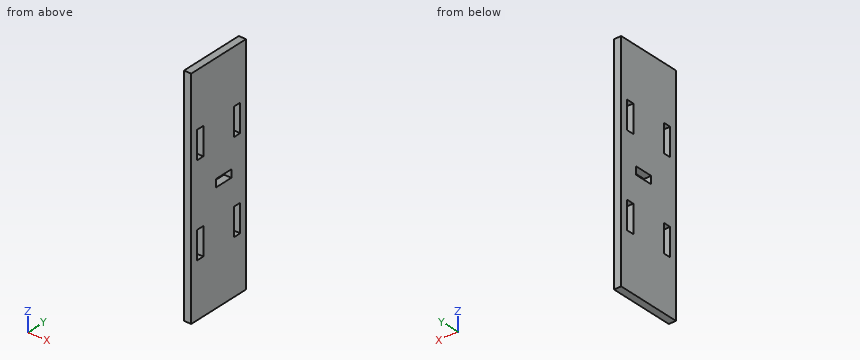
from build123d import *

# Parameters (mm, degrees)
SKETCH1_W           = 685
SKETCH1_H           = 250
BASE_FLANGE1_DEPTH  = 8
SKETCH6_W           = 60
SKETCH6_H           = 8
SKETCH6_W_2         = 70
EXTRUDE1_DEPTH      = 8
SKETCH7_W           = 250
SKETCH7_H           = 73.5
BASE_FLANGE2_DEPTH  = 8
SKETCH12_W          = 30.5
SKETCH12_H          = 8.5
EXTRUDE2_DEPTH      = 699.681794525
SKETCH14_W          = 250
SKETCH14_H          = 8
BASE_FLANGE3_DEPTH  = 50.5
SKETCH19_W          = 60
SKETCH19_H          = 8
SKETCH19_W_2        = 70
EXTRUDE3_DEPTH      = 8
BREAK_CORNER1_START = 41.5
BREAK_CORNER1_DEPTH = 8
EXTRUDE4_DEPTH      = 8
BASE_FLANGE4_DEPTH  = 8
SKETCH38_W          = 8.5
SKETCH38_H          = 20.5
EXTRUDE5_DEPTH      = 10
SKETCH39_W          = 20.5
SKETCH39_H          = 8.5
EXTRUDE6_DEPTH      = 10


# Read off the part's stored shape, not the designer's step: Break-Corner1
# Sheet-metal steps are written as plain solids
with BuildPart() as part:
    # Sketch1 → Base-Flange1 (new body)
    with BuildSketch(Plane(origin=(0, 0, 0), x_dir=(1, 0, 0), z_dir=(0, 1, 0))):
        Rectangle(SKETCH1_W, SKETCH1_H)
    extrude(amount=-BASE_FLANGE1_DEPTH)

    # Sketch6 → Extrude1 (cut)
    with BuildSketch(Plane(origin=(342.5, 0, 0), x_dir=(0, 0, -1), z_dir=(1, 0, 0))):
        with Locations((-95, -4)):
            Rectangle(SKETCH6_W, SKETCH6_H)
        with Locations((95, -4)):
            Rectangle(SKETCH6_W, SKETCH6_H)
        with Locations((0, -4)):
            Rectangle(SKETCH6_W_2, SKETCH6_H)
    extrude1 = extrude(amount=-EXTRUDE1_DEPTH, mode=Mode.SUBTRACT)

    # Mirror1: Extrude1 across plane
    add(extrude1.mirror(Plane(origin=(0, 0, 0), x_dir=(0, 0, 1), z_dir=(1, 0, 0))), mode=Mode.SUBTRACT)

    # Sketch39 → Extrude6 (cut)
    with BuildSketch(Plane.XZ.offset(8)):
        with Locations((289.5, 0)):
            Rectangle(SKETCH39_W, SKETCH39_H)
        with Locations((229.5, 0)):
            Rectangle(SKETCH39_W, SKETCH39_H)
        with Locations((-289.5, 0)):
            Rectangle(SKETCH39_W, SKETCH39_H)
        with Locations((-229.5, 0)):
            Rectangle(SKETCH39_W, SKETCH39_H)
    extrude(amount=-EXTRUDE6_DEPTH, mode=Mode.SUBTRACT)


with BuildPart() as body_2:
    # Sketch7 → Base-Flange2 (new body)
    with BuildSketch(Plane(origin=(334.5, 0, 0), x_dir=(0, 0, -1), z_dir=(1, 0, 0))):
        with Locations((0, 20.75)):
            Rectangle(SKETCH7_W, SKETCH7_H)
    extrude(amount=BASE_FLANGE2_DEPTH)

    # Sketch12 → Extrude2 (cut, through all)
    with BuildSketch(Plane(origin=(342.5, 0, 0), x_dir=(0, 0, -1), z_dir=(1, 0, 0))):
        with Locations((-50, -4)):
            Rectangle(SKETCH12_W, SKETCH12_H)
        with Locations((50, -4)):
            Rectangle(SKETCH12_W, SKETCH12_H)
        with Locations((50, 45.5)):
            Rectangle(SKETCH12_W, SKETCH12_H)
        with Locations((-50, 45.5)):
            Rectangle(SKETCH12_W, SKETCH12_H)
    extrude(amount=-EXTRUDE2_DEPTH, mode=Mode.SUBTRACT)

    # Sketch38 → Extrude5 (cut)
    with BuildSketch(Plane(origin=(342.5, 0, 0), x_dir=(0, 0, -1), z_dir=(1, 0, 0))):
        with Locations((0, 27.5)):
            Rectangle(SKETCH38_W, SKETCH38_H)
    extrude(amount=-EXTRUDE5_DEPTH, mode=Mode.SUBTRACT)


with BuildPart() as body_3:
    # Sketch14 → Base-Flange3 (new body)
    with BuildSketch(Plane.ZY.offset(-334.5)):
        with Locations((0, 45.5)):
            Rectangle(SKETCH14_W, SKETCH14_H)
    extrude(amount=-BASE_FLANGE3_DEPTH)

    # Sketch19 → Extrude3 (cut)
    with BuildSketch(Plane(origin=(342.5, 0, 0), x_dir=(0, 0, -1), z_dir=(1, 0, 0))):
        with Locations((95, 45.5)):
            Rectangle(SKETCH19_W, SKETCH19_H)
        with Locations((0, 45.5)):
            Rectangle(SKETCH19_W_2, SKETCH19_H)
        with Locations((-95, 45.5)):
            Rectangle(SKETCH19_W, SKETCH19_H)
    extrude(amount=-EXTRUDE3_DEPTH, mode=Mode.SUBTRACT)

    # Break-Corner1 outline → Break-Corner1 (cut)
    with BuildSketch(Plane(origin=(0, 0, 0), x_dir=(1, 0, 0), z_dir=(0, 1, 0)).offset(BREAK_CORNER1_START)):
        Polygon((385, -125), (385, -110), (370, -125), align=None)
        Polygon((370, 125), (385, 110), (385, 125), align=None)
    extrude(amount=BREAK_CORNER1_DEPTH, mode=Mode.SUBTRACT)

    # Sketch20 → Extrude4 (cut)
    with BuildSketch(Plane(origin=(0, 49.5, 0), x_dir=(1, 0, 0), z_dir=(0, 1, 0))):
        with BuildLine():
            Line((367, 75), (367, 55))
            ThreePointArc((367, 55), (362.5, 50.5), (358, 55))
            Line((358, 55), (358, 75))
            ThreePointArc((358, 75), (362.5, 79.5), (367, 75))
        make_face()
        with BuildLine():
            Line((367, -75), (367, -55))
            ThreePointArc((367, -55), (362.5, -50.5), (358, -55))
            Line((358, -55), (358, -75))
            ThreePointArc((358, -75), (362.5, -79.5), (367, -75))
        make_face()
    extrude(amount=-EXTRUDE4_DEPTH, mode=Mode.SUBTRACT)


with BuildPart() as body_4:
    # Mirror4: mirrored copy
    add(body_3.part.mirror(Plane(origin=(0, 0, 0), x_dir=(0, 0, 1), z_dir=(1, 0, 0))))


with BuildPart() as body_5:
    # Sketch29 → Base-Flange4 (new body)
    with BuildSketch(Plane.XY.offset(4)):
        Polygon((219.5, 0), (219.5, -8), (239.5, -8), (239.5, 0), (279.5, 0), (279.5, -8), (299.5, -8), (299.5, 0), (334.5, 0), (334.5, 17.5), (342.5, 17.5), (342.5, 37.5), (334.5, 37.5), (334.5, 57.5), (194.5, 10), (194.5, 0), align=None)
    extrude(amount=-BASE_FLANGE4_DEPTH)


with BuildPart() as body_6:
    # Mirror5: mirrored copy
    add(body_5.part.mirror(Plane(origin=(0, 0, 0), x_dir=(0, 0, 1), z_dir=(1, 0, 0))))


with BuildPart() as body_7:
    # Mirror3: mirrored copy
    add(body_2.part.mirror(Plane(origin=(0, 0, 0), x_dir=(0, 0, 1), z_dir=(1, 0, 0))))


solid = body_7.part
Check sheet for the modelled part. Datum: model origin and axes. Units: mm. Round coordinates to 2 decimals unless told otherwise and drop trailing zeros. Loops run counter-clockwise (first coordinate to the right, second up) from the corner with the lowest first, then second, coordinate; pieces in that order, holes last. Notation, with made-up numbers: (-16, 7.5) - (-6, 7.5) arc R24 ccw to (-6, 36.5) - close; hole circle Ø6 at (44, -38.75). An arc over 180 degrees is marked (long way). Answer as CSV lines item,"result". Start each with the question number.
Item 1: Section check C-C (x = -340.75). Record the boundary of the cut face in (y, z).
Item 2: Scan lines: line 1 (Z direction, x = -341.25, y = 45.5); line 2 (Y direction, x = -335, z = 45); line 3 (Z direction, x = -340.25, y = 21). Record each from-to range of solid material in increasing order. Write a range as [from, to].
Item 3: Section check B-B (y = 44.5). Record the boundary of the cut face in (x, z), and give its area (3 significant figures).
Item 4: Section check A-A (z = 40). Record the boundary of the cut face in (x, y), and give its area (3 significant figures).
Report:
1,outline,"(-16, -125) - (57.5, -125) - (57.5, 125) - (-16, 125) - close; hole (-8.25, -65.25) - (0.25, -65.25) - (0.25, -34.75) - (-8.25, -34.75) - close; hole (-8.25, 34.75) - (0.25, 34.75) - (0.25, 65.25) - (-8.25, 65.25) - close; hole (17.25, -4.25) - (37.75, -4.25) - (37.75, 4.25) - (17.25, 4.25) - close; hole (41.25, -65.25) - (49.75, -65.25) - (49.75, -34.75) - (41.25, -34.75) - close; hole (41.25, 34.75) - (49.75, 34.75) - (49.75, 65.25) - (41.25, 65.25) - close"
2,line 1,"z = [-125, -65.25], [-34.75, 34.75], [65.25, 125]"
2,line 2,"y = [-16, -8.25], [0.25, 41.25], [49.75, 57.5]"
2,line 3,"z = [-125, -4.25], [4.25, 125]"
3,outline,"(-342.5, -125) - (-334.5, -125) - (-334.5, -65.25) - (-342.5, -65.25) - close; (-342.5, -34.75) - (-334.5, -34.75) - (-334.5, 34.75) - (-342.5, 34.75) - close; (-342.5, 65.25) - (-334.5, 65.25) - (-334.5, 125) - (-342.5, 125) - close"
3,area,"1,510 mm2"
4,outline,"(-342.5, -16) - (-334.5, -16) - (-334.5, -8.25) - (-342.5, -8.25) - close; (-342.5, 0.25) - (-334.5, 0.25) - (-334.5, 41.25) - (-342.5, 41.25) - close; (-342.5, 49.75) - (-334.5, 49.75) - (-334.5, 57.5) - (-342.5, 57.5) - close"
4,area,"452 mm2"
